Geometry: final body of the model. Coordinates: model frame, mm. A direction names the side the tool comes from. Round coordinates to 2 decimals unless told otherwise and drop trailing zeros. Loops run counter-clockwise (first coordinate to the right, second up) from the corner with the lowest first, then second, coordinate; pieces in that order, holes last. Notation, with made-up numbers: (83.25, 7) - (116.25, 7) arc R24 cw to (116.25, 31) - close; hole circle Ø7 at (72, 66). An arc over 180 degrees is marked (long way). Return JSON: item names as keys, results as strings. Group by question number.
1. Section B-B on x = -6.5. Return loops of the section in (y, z) (3 decimals), and give its area (3 significant figures).
2. Set-up query: faces 4 (the face through (-23, 4, -7)), 5 (the face through (-0.18, 12.03, 16.82)), 6 (the face through (20, 9, -13.575)). Return all of +Z, -Z, +X, -X, +Y, -Y with unobstructed straight access to the full face (end or side cutting, diameter ignored); none if empty.
3. Section A-A on x = 0. Return loops of the section in (y, z) (3 decimals), and give its area (3 significant figures).
4. Section C-C on y = 49. Return loops of the section in (x, z) (3 decimals), and give its area (3 significant figures).
5. Section D-D on y = 40.7. Return loops of the section in (x, z) (3 decimals), and give its area (3 significant figures).
6. Draft query along X for faces 1 (the face through (-21, 14, 7)), 2 (the face through (20, 9, 17.125)), 3 (the face through (-10.467, 15.274, -24.358)). Return one class per face: +X half, -X half, draft (parallel to the pull), parting line (faces both ways), or undercut.
7. First-contact query: pin 1 Ø2.5 at (x, y) = (10.25, 16.25) entering from +Z (3 decimals); pin 2 Ø11 at (x, z) = (3.5, 22) entering from +Y; pin 3 Ø4 at (x, z) = (22, -7) entering from +Y; pin 4 Ø8 at (x, z) = (-5, -5.5) entering from -Y. Flat tips, straight axial feed; report the tip coordinate or a pass-through.
8. Material intervals for probe 1 along X at (y, z) = (27, -7.5); probe 2 along Z at (x, y) = (19.5, 8.5) (3 decimals); probe 3 along Y at (x, z) = (-10.25, -25.1) (3 decimals), sorted ascending.
from build123d import *

# Parameters (mm, degrees)
SKETCH1_W               = 50
SKETCH1_H               = 58.25
BOSS_EXTRUDE1_DEPTH     = 10
SKETCH2_R               = 2.15
CUT_EXTRUDE1_DEPTH      = 4
SKETCH5_W               = 25
SKETCH5_H               = 6
BOSS_EXTRUDE3_DEPTH     = 46
CUT_EXTRUDE3_REACH      = 86.582
SKETCH6_W               = 22
SKETCH6_H               = 19.25
SKETCH7_R               = 1
CUT_EXTRUDE4_DEPTH      = 2.5
CUT_EXTRUDE5_REACH      = 84.21
SKETCH8_R               = 2
BOSS_EXTRUDE4_DEPTH     = 5
CHAMFER1_SIZE           = 7.5
CHAMFER2_SIZE           = 10
CHAMFER4_SIZE           = 15
CHAMFER5_SIZE           = 5
CHAMFER7_SIZE           = 2
CUT_EXTRUDE6_REACH      = 86.582
SKETCH10_R              = 3.1
CHAMFER8_SIZE           = 1
BOSS_EXTRUDE5_REACH     = 75.42
CUT_EXTRUDE12_REACH     = 78.095
SKETCH17_W              = 10
SKETCH17_H              = 13.5
LPATTERN1_COUNT         = 2
LPATTERN1_PITCH         = 30.7
MIRROR3_COPY_1_REACH    = 78.095
MIRROR3_COPY_1_SKETCH_W = 10
MIRROR3_COPY_1_SKETCH_H = 13.5


# Some blends are built 0.0001 mm under size
with BuildPart() as part:
    # Sketch1 → Boss-Extrude1 (new body)
    with BuildSketch(Plane(origin=(0, 0, 0), x_dir=(1, 0, 0), z_dir=(0, 1, 0))):
        Rectangle(SKETCH1_W, SKETCH1_H)
    extrude(amount=BOSS_EXTRUDE1_DEPTH)

    # Sketch2 → Cut-Extrude1 (cut)
    with BuildSketch(Plane(origin=(0, 0, 0), x_dir=(1, 0, 0), z_dir=(0, 1, 0))):
        with Locations(Location((-21, 8.575, 0), (0, 0, 270))):
            Circle(SKETCH2_R)
        with Locations(Location((-21, -22.125, 0), (0, 0, 270))):
            Circle(SKETCH2_R)
        with Locations(Location((21, 8.575, 0), (0, 0, 270))):
            Circle(SKETCH2_R)
        with Locations(Location((21, -22.125, 0), (0, 0, 270))):
            Circle(SKETCH2_R)
    extrude(amount=CUT_EXTRUDE1_DEPTH, mode=Mode.SUBTRACT)

    # Sketch5 → Boss-Extrude3 (add)
    with BuildSketch(Plane(origin=(0, 10, 0), x_dir=(1, 0, 0), z_dir=(0, 1, 0))):
        with Locations((0, 26.125)):
            Rectangle(SKETCH5_W, SKETCH5_H)
    extrude(amount=BOSS_EXTRUDE3_DEPTH)

    # Sketch6 → Cut-Extrude3 (cut, up to next)
    with BuildSketch(Plane(origin=(0, 0, -29.125), x_dir=(-1, 0, 0), z_dir=(0, 0, -1)), mode=Mode.PRIVATE) as cut_extrude3_sk1:
        with Locations((0, 28.625)):
            Rectangle(SKETCH6_W, SKETCH6_H)
    cut_extrude3_tool1 = extrude(cut_extrude3_sk1.sketch, amount=-CUT_EXTRUDE3_REACH, mode=Mode.PRIVATE) & part.part
    add(cut_extrude3_tool1.solids().sort_by_distance((0, 28.625, -29.125))[0], mode=Mode.SUBTRACT)

    # Sketch7 → Cut-Extrude4 (cut)
    with BuildSketch(Plane.XY.offset(-23.125)):
        with Locations((10.25, 16.25)):
            Circle(SKETCH7_R)
        with Locations((-10.25, 16.25)):
            Circle(SKETCH7_R)
        with Locations((-10.25, 40.7)):
            Circle(SKETCH7_R)
        with Locations((10.25, 40.7)):
            Circle(SKETCH7_R)
    extrude(amount=-CUT_EXTRUDE4_DEPTH, mode=Mode.SUBTRACT)

    # Sketch8 → Cut-Extrude5 (cut, up to next)
    with BuildSketch(Plane.XY.offset(-25.625), mode=Mode.PRIVATE) as cut_extrude5_sk1:
        with Locations((-10.25, 40.7)):
            Circle(SKETCH8_R)
    cut_extrude5_tool1 = extrude(cut_extrude5_sk1.sketch, amount=-CUT_EXTRUDE5_REACH, mode=Mode.PRIVATE) & part.part
    # Sketch8 → Cut-Extrude5 (cut, up to next)
    with BuildSketch(Plane.XY.offset(-25.625), mode=Mode.PRIVATE) as cut_extrude5_sk2:
        with Locations((10.25, 40.7)):
            Circle(SKETCH8_R)
    cut_extrude5_tool2 = extrude(cut_extrude5_sk2.sketch, amount=-CUT_EXTRUDE5_REACH, mode=Mode.PRIVATE) & part.part
    # Sketch8 → Cut-Extrude5 (cut, up to next)
    with BuildSketch(Plane.XY.offset(-25.625), mode=Mode.PRIVATE) as cut_extrude5_sk3:
        with Locations((10.25, 16.25)):
            Circle(SKETCH8_R)
    cut_extrude5_tool3 = extrude(cut_extrude5_sk3.sketch, amount=-CUT_EXTRUDE5_REACH, mode=Mode.PRIVATE) & part.part
    # Sketch8 → Cut-Extrude5 (cut, up to next)
    with BuildSketch(Plane.XY.offset(-25.625), mode=Mode.PRIVATE) as cut_extrude5_sk4:
        with Locations((-10.25, 16.25)):
            Circle(SKETCH8_R)
    cut_extrude5_tool4 = extrude(cut_extrude5_sk4.sketch, amount=-CUT_EXTRUDE5_REACH, mode=Mode.PRIVATE) & part.part
    add(cut_extrude5_tool1.solids().sort_by_distance((-10.25, 40.7, -25.625))[0], mode=Mode.SUBTRACT)
    add(cut_extrude5_tool2.solids().sort_by_distance((10.25, 40.7, -25.625))[0], mode=Mode.SUBTRACT)
    add(cut_extrude5_tool3.solids().sort_by_distance((10.25, 16.25, -25.625))[0], mode=Mode.SUBTRACT)
    add(cut_extrude5_tool4.solids().sort_by_distance((-10.25, 16.25, -25.625))[0], mode=Mode.SUBTRACT)

    # Sketch9 → Boss-Extrude4 (add)
    with BuildSketch(Plane(origin=(12.5, 0, 0), x_dir=(0, 0, -1), z_dir=(1, 0, 0))):
        Polygon((29.125, 56), (23.125, 56), (-29.125, 10), (29.125, 10), align=None)
    boss_extrude4 = extrude(amount=BOSS_EXTRUDE4_DEPTH)

    # Mirror1: Boss-Extrude4 across plane
    add(boss_extrude4.mirror(Plane(origin=(0, 0, 0), x_dir=(0, 0, 1), z_dir=(1, 0, 0))))

    # Chamfer1
    chamfer1_edges = [part.edges().sort_by_distance(p)[0] for p in [
        (17.5, 10, 0),
        (-17.5, 10, 0),
    ]]
    chamfer(chamfer1_edges, length=CHAMFER1_SIZE - 0.0001)  # a hair under: the kernel refuses the full size

    # Chamfer2
    chamfer2_edges = [part.edges().sort_by_distance(p)[0] for p in [
        (-25, 5, -29.125),
        (25, 5, -29.125),
    ]]
    chamfer(chamfer2_edges, length=CHAMFER2_SIZE)

    # Chamfer4
    # the kernel refuses this chamfer: 15 mm, written as the material it takes off along each edge
    with BuildSketch(Plane(origin=(-53.575244819, 0, -29.125), x_dir=(0, 0.9996219169112968, -0.02749587661058632), z_dir=(1, 0, 0))) as chamfer4_piece_1:
        Polygon((CHAMFER4_SIZE * 0.999621916911, CHAMFER4_SIZE * 0.0274958766106), (-CHAMFER4_SIZE * 0.0274958766106, CHAMFER4_SIZE * 0.999621916911), (0, 0), align=None)
    extrude(amount=107.150489639, mode=Mode.SUBTRACT)

    # Chamfer5
    chamfer5_edges = [part.edges().sort_by_distance(p)[0] for p in [
        (17.5, 56, -24.875),
        (-17.5, 56, -24.875),
    ]]
    chamfer(chamfer5_edges, length=CHAMFER5_SIZE)

    # Chamfer7
    chamfer7_edges = [part.edges().sort_by_distance(p)[0] for p in [
        (-11, 38.25, -26.125),
        (-11, 19, -26.125),
        (11, 19, -26.125),
        (11, 38.25, -26.125),
    ]]
    chamfer(chamfer7_edges, length=CHAMFER7_SIZE)

    # Sketch10 → Cut-Extrude6 (cut, up to next)
    with BuildSketch(Plane(origin=(0, 0, -29.125), x_dir=(-1, 0, 0), z_dir=(0, 0, -1)), mode=Mode.PRIVATE) as cut_extrude6_sk1:
        with Locations((0, 49)):
            Circle(SKETCH10_R)
    cut_extrude6_tool1 = extrude(cut_extrude6_sk1.sketch, amount=-CUT_EXTRUDE6_REACH, mode=Mode.PRIVATE) & part.part
    add(cut_extrude6_tool1.solids().sort_by_distance((0, 49, -29.125))[0], mode=Mode.SUBTRACT)

    # Chamfer8
    chamfer8_edges = [part.edges().sort_by_distance(p)[0] for p in [
        (3.1, 49, -29.125),
        (3.1, 49, -23.125),
    ]]
    chamfer(chamfer8_edges, length=CHAMFER8_SIZE)

    # Sketch11 → Boss-Extrude5 (add, up to next)
    with BuildSketch(Plane(origin=(-12.5, 0, 0), x_dir=(0, 0, -1), z_dir=(1, 0, 0)), mode=Mode.PRIVATE) as boss_extrude5_sk1:
        Polygon((-19.125, 10), (23.125, 10), (23.125, 14), (-14.581521739, 14), align=None)
    boss_extrude5_tool1 = extrude(boss_extrude5_sk1.sketch, amount=BOSS_EXTRUDE5_REACH, mode=Mode.PRIVATE) - part.part
    add(boss_extrude5_tool1.solids().sort_by_distance((-12.5, 11.962117, -3.114355))[0])

    # Sketch17 → Cut-Extrude12 (cut, up to next)
    with BuildSketch(Plane(origin=(17.5, 0, 0), x_dir=(0, 0, -1), z_dir=(1, 0, 0)), mode=Mode.PRIVATE) as cut_extrude12_sk1:
        with Locations((8.575, 10.75)):
            Rectangle(SKETCH17_W, SKETCH17_H)
    cut_extrude12_tool1 = extrude(cut_extrude12_sk1.sketch, amount=CUT_EXTRUDE12_REACH, mode=Mode.PRIVATE) & part.part
    cut_extrude12 = cut_extrude12_tool1.solids().sort_by_distance((17.5, 10.75, -8.575))[0]
    add(cut_extrude12, mode=Mode.SUBTRACT)

    # LPattern1: Cut-Extrude12 ×2
    with Locations(*[(0, 0, i * LPATTERN1_PITCH) for i in range(1, LPATTERN1_COUNT)]):
        add(cut_extrude12, mode=Mode.SUBTRACT)

    # Mirror3: Cut-Extrude12 across plane
    add(cut_extrude12.mirror(Plane(origin=(0, 0, 0), x_dir=(0, 0, 1), z_dir=(1, 0, 0))), mode=Mode.SUBTRACT)

    # Mirror3 copy 1 sketch → Mirror3 copy 1 (cut, up to next)
    with BuildSketch(Plane(origin=(-17.5, 0, 30.7), x_dir=(0, 0, -1), z_dir=(-1, 0, 0)), mode=Mode.PRIVATE) as mirror3_copy_1_sk1:
        with Locations((8.575, -10.75)):
            Rectangle(MIRROR3_COPY_1_SKETCH_W, MIRROR3_COPY_1_SKETCH_H)
    mirror3_copy_1_tool1 = extrude(mirror3_copy_1_sk1.sketch, amount=MIRROR3_COPY_1_REACH, mode=Mode.PRIVATE) & part.part
    add(mirror3_copy_1_tool1.solids().sort_by_distance((-17.5, 10.75, 22.125))[0], mode=Mode.SUBTRACT)


solid = part.part
Taken from the geometry:
{
 "1": {"outline": "(0, -14.125) - (15, -29.125) - (19, -29.125) - (19, -23.125) - (14, -23.125) - (14, 14.582) - (10, 19.125) - (10, 29.125) - (0, 29.125) - close; (38.25, -29.125) - (56, -29.125) - (56, -23.125) - (38.25, -23.125) - close", "area": "790 mm2"},
 "2": {"face 4": "-X, +Y", "face 5": "+Z, +Y", "face 6": "+X, +Y"},
 "3": {"outline": "(0, -14.125) - (15, -29.125) - (19, -29.125) - (19, -23.125) - (14, -23.125) - (14, 14.582) - (10, 19.125) - (10, 29.125) - (0, 29.125) - close; (38.25, -29.125) - (44.9, -29.125) - (45.9, -28.125) - (45.9, -24.125) - (44.9, -23.125) - (38.25, -23.125) - close; (52.1, -28.125) - (53.1, -29.125) - (56, -29.125) - (56, -23.125) - (53.1, -23.125) - (52.1, -24.125) - close", "area": "751 mm2"},
 "4": {"outline": "(-17.5, -26.625) - (-15, -29.125) - (-4.1, -29.125) - (-3.1, -28.125) - (-3.1, -24.125) - (-4.1, -23.125) - (-12.5, -23.125) - (-12.5, -15.174) - (-17.5, -15.174) - close; (3.1, -28.125) - (4.1, -29.125) - (15, -29.125) - (17.5, -26.625) - (17.5, -15.174) - (12.5, -15.174) - (12.5, -23.125) - (4.1, -23.125) - (3.1, -24.125) - close", "area": "244 mm2"},
 "5": {"outline": "(-17.5, -26.625) - (-15, -29.125) - (-12.25, -29.125) - (-12.25, -25.625) - (-11.25, -25.625) - (-11.25, -23.125) - (-12.5, -23.125) - (-12.5, -5.746) - (-17.5, -5.746) - close; (-9.25, -25.625) - (-8.25, -25.625) - (-8.25, -29.125) - (8.25, -29.125) - (8.25, -25.625) - (9.25, -25.625) - (9.25, -23.125) - (-9.25, -23.125) - close; (11.25, -25.625) - (12.25, -25.625) - (12.25, -29.125) - (15, -29.125) - (17.5, -26.625) - (17.5, -5.746) - (12.5, -5.746) - (12.5, -23.125) - (11.25, -23.125) - close", "area": "340 mm2"},
 "6": {"face 1": "-X half", "face 2": "draft", "face 3": "undercut"},
 "7": {"pin 1": "z = -23.125", "pin 2": "y = 12.31", "pin 3": "y = 4", "pin 4": "y = 0"},
 "8": {"probe 1": "-17.5 to -12.5, 12.5 to 17.5", "probe 2": "-22.625 to -13.575, -3.575 to 17.125, 27.125 to 29.125", "probe 3": "10.975 to 15.25, 17.25 to 20.25, 37 to 39.7, 41.7 to 56"}
}
